Geometry check sheet. Reference: the model listing, model coordinates, mm. A direction names the side the tool comes from. Coordinates: 2 decimals unless noted, no trailing zeros. Order: outer loops, then holes, each group sorted by start corner. A loop starts at its lowest first (then second) coordinate and runs counter-clockwise, first axis right, second up. Notation, with made-up numbers: (47.5, 5) - (51.5, 5) arc R6 cw to (51.5, 11) - close; hole circle Ø10 at (70, 77.25). An arc over 180 degrees is marked (long way). Return JSON: item names as keys, results as strings. Group by question number.
Item 1: Section check B-B on y = 0.5. Enter the section's corners in (x, z).
Item 2: Section check A-A on z = 10.75. Enter the section's corners in (x, y).
Item 3: Section check D-D on z = 3. Enter the section's corners in (x, y), then the cut area to 3 significant figures.
Item 4: Section check C-C on x = 0. Enter the section's corners in (y, z).
Item 5: Draft check along X on faces 3 (the flat face through (-1.11, -3.32, 6.9)), 4 (the flat face through (1.11, 3.32, 6.9)), 5 (the flat face through (-0.822, -2.467, 8.774)), 6 (the cylindrical face through (0.75, 0.03, 1.68)). Enter one of: pulls with the +X half, pulls with the -X half, needs draft (parallel to the pull), parting line crosses it, or undercut.
Item 6: Scan lines: probe 1 along Y at (x, z) = (0.5, 5.5); probe 2 along Y at (x, z) = (2, 10.5); probe 3 along X at (y, z) = (-0.5, 10). Record each from-to range of solid material in increasing order.
Item 7: Gauge pin test, flat ends, axial feed: pin 1 (3 mm diameter, centred on x = -3, z = 7, fed in from +Y); pin 2 (2 mm diameter, centred on x = -2, z = 7.5, fed in from -Y); pin 3 (1 mm diameter, centred on x = 2.5, z = 4.5, fed in from +Y). Record the tip position at first contact, or that the pin passes through.
Item 8: Tool access check on faces 1 (the flat face through (-2.32, 2.62, 6.9)), 2 (the flat face through (2.547, 0.522, 8.774)). Record the directions out of +Z, -Z, +X, -X, +Y, -Y that give a thin tool (end or side, any length) a straight path to the whole face; none if there is none.
from build123d import *

# Parameters (mm, degrees)
RESSALTO_EXTRUS_O1_DEPTH = 14
CORTE_EXTRUS_O1_DEPTH    = 10.6
CORTE_EXTRUS_O2_REACH    = 17.047
ESBO_O3_R                = 0.75


with BuildPart() as part:
    # Esboço1 → Ressalto-extrusão1 (new body)
    with BuildSketch(Plane.XY):
        Polygon((-0.842772028, 3.952602768), (-3.844440422, 1.246439398), (-3.001668394, -2.70616337), (0.842772028, -3.952602768), (3.844440422, -1.246439398), (3.001668394, 2.70616337), align=None)
    extrude(amount=RESSALTO_EXTRUS_O1_DEPTH)

    # Esboço2 → Corte-extrusão1 (cut)
    with BuildSketch(Plane.XY.offset(14)):
        Polygon((2.229810807, 2.010292789), (-0.626059221, 2.936219199), (-2.855870028, 0.92592641), (-2.229810807, -2.010292789), (0.626059221, -2.936219199), (2.855870028, -0.92592641), align=None)
    extrude(amount=-CORTE_EXTRUS_O1_DEPTH, mode=Mode.SUBTRACT)

    # Esboço3 → Corte-extrusão2 (cut, up to next)
    with BuildSketch(Plane(origin=(0, 0, 0), x_dir=(-1, 0, 0), z_dir=(0, 0, -1)), mode=Mode.PRIVATE) as corte_extrus_o2_sk1:
        Circle(ESBO_O3_R)
    corte_extrus_o2_tool1 = extrude(corte_extrus_o2_sk1.sketch, amount=-CORTE_EXTRUS_O2_REACH, mode=Mode.PRIVATE) & part.part
    add(corte_extrus_o2_tool1.solids().sort_by_distance((0, 0, 0))[0], mode=Mode.SUBTRACT)


solid = part.part
Computed:
{
 "1": {"outline": "(-3.69, 0) - (-0.56, 0) - (-0.56, 3.4) - (-2.77, 3.4) - (-2.77, 14) - (-3.69, 14) - close; (0.56, 0) - (3.47, 0) - (3.47, 14) - (2.55, 14) - (2.55, 3.4) - (0.56, 3.4) - close"},
 "2": {"outline": "(-3.84, 1.25) - (-3, -2.71) - (0.84, -3.95) - (3.84, -1.25) - (3, 2.71) - (-0.84, 3.95) - close; hole (-2.86, 0.93) - (-2.23, -2.01) - (0.63, -2.94) - (2.86, -0.93) - (2.23, 2.01) - (-0.63, 2.94) - close"},
 "3": {"outline": "(-3.84, 1.25) - (-3, -2.71) - (0.84, -3.95) - (3.84, -1.25) - (3, 2.71) - (-0.84, 3.95) - close; hole circle Ø1.5 at (0, 0)", "area": "40.7 mm²"},
 "4": {"outline": "(-3.68, 0) - (-0.75, 0) - (-0.75, 3.4) - (-2.73, 3.4) - (-2.73, 14) - (-3.68, 14) - close; (0.75, 0) - (3.68, 0) - (3.68, 14) - (2.73, 14) - (2.73, 3.4) - (0.75, 3.4) - close"},
 "5": {"face 3": "pulls with the -X half", "face 4": "pulls with the +X half", "face 5": "undercut", "face 6": "undercut"},
 "6": {"probe 1": "y = -3.84 to -2.9, 2.57 to 3.52", "probe 2": "y = -2.91 to -1.7, 2.08 to 3.03", "probe 3": "x = -3.47 to -2.55, 2.77 to 3.69"},
 "7": {"pin 1": "stops at y = 3.36", "pin 2": "stops at y = -3.36", "pin 3": "stops at y = 3.03"},
 "8": {"face 1": "+Z, -Z, -X, +Y", "face 2": "+Z"}
}
